Can you work these out from the model? Positions are in its coordinate system, mm. A direction names the side the tool comes from. Coordinates: 2 decimals unless noted, no trailing zeros. Loops run counter-clockwise (first coordinate to the right, second up) from the corner with the lowest first, then second, coordinate; pieces in that order, holes last. Notation, with made-up numbers: (34, -22.75) -> (60, -22.75) arc R17 cw to (60, -14.75) -> close; hole circle Ø11 at (74.5, 62). An arc over 180 degrees is marked (long way). Put each result on its own line as item: value. Start each with the question number.
Item 1: Will these pins go through, and if not, where does the flat tip stop? P1, Ø1.5, axis at y = 5, z = -3, coming from the +X side; P2, Ø2.5, axis at x = 3, y = 5, coming from the +Z side; P3, Ø1, axis at x = 3.5, y = 4, coming from the -Z side.
Item 2: If we section it at D-D on z = -3.25: Please give me the cut outline in (x, y).
Item 3: If we section it at C-C on x = 0: Please give me the cut outline in (y, z), plus the area to 3 significant figures.
Item 4: For faces 1 (the flat face through (-4.3, 5, -3)), 2 (the flat face through (0, 4, 5)), 3 (the flat face through (-3.5, 7, -3.5)), 4 (the flat face through (4.3, 5, -3)), 5 (the flat face through (0, 4, -5)), which set-ups out of +Z, -Z, +X, -X, +Y, -Y let a thin tool reach every point of the face, with its end or its side?
Item 5: We'd pull the mould along Z, two halves only. Please class faces 6 (the flat face through (-5, 4, 0)), 7 (the flat face through (3, 5, -4.3)), 8 (the cylindrical face through (5.723, 1.972, -1.802)), 9 (the cylindrical face through (5, 2, 1)): pulls with the +Z half, pulls with the -Z half, needs draft (parallel to the pull), parting line crosses it, or undercut.
Item 6: If we section it at A-A on z = 0: Please give me the cut outline in (x, y).
Item 7: Please list where these lines run through material, in increasing order: L1, parallel to Y at x = -5.7, z = 0; L2, parallel to Z at x = 0, y = 1.6; L3, parallel to Y at x = 0.75, z = -5.25. Write a range as from..to.
Item 8: If we section it at B-B on y = 5: Please give me the cut outline in (x, z).
```python
from build123d import *

# Parameters (mm, degrees)
SKETCH1_R               = 6
SKETCH1_R_2             = 4.5
BOSS_EXTRUDE5_DEPTH     = 4
BOSS_EXTRUDE6_DEPTH     = 3
SKETCH4_R               = 1
CUT_EXTRUDE1_DEPTH      = 7
CUT_EXTRUDE1_DEPTH_BACK = 7


with BuildPart() as part:
    # Sketch1 → Boss-Extrude5 (new body)
    with BuildSketch(Plane(origin=(0, 0, 0), x_dir=(1, 0, 0), z_dir=(0, 1, 0))):
        Circle(SKETCH1_R)
        Circle(SKETCH1_R_2, mode=Mode.SUBTRACT)
    extrude(amount=BOSS_EXTRUDE5_DEPTH)

    # Sketch3 → Boss-Extrude6 (add)
    with BuildSketch(Plane(origin=(0, 4, 0), x_dir=(1, 0, 0), z_dir=(0, 1, 0))):
        with BuildLine():
            Line((1.326649916, 4.3), (4.3, 4.3))
            Line((4.3, 4.3), (4.3, 1.326649916))
            ThreePointArc((4.3, 1.326649916), (3.181980515, 3.181980515), (1.326649916, 4.3))
        make_face()
        with BuildLine():
            Line((-4.3, -4.3), (-1.326649916, -4.3))
            ThreePointArc((-1.326649916, -4.3), (-3.181980515, -3.181980515), (-4.3, -1.326649916))
            Line((-4.3, -1.326649916), (-4.3, -4.3))
        make_face()
        with BuildLine():
            Line((-4.3, 4.3), (-1.326649916, 4.3))
            ThreePointArc((-1.326649916, 4.3), (-3.181980515, 3.181980515), (-4.3, 1.326649916))
            Line((-4.3, 1.326649916), (-4.3, 4.3))
        make_face()
        with BuildLine():
            Line((4.3, -4.3), (4.3, -1.326649916))
            ThreePointArc((4.3, -1.326649916), (3.181980515, -3.181980515), (1.326649916, -4.3))
            Line((1.326649916, -4.3), (4.3, -4.3))
        make_face()
    extrude(amount=BOSS_EXTRUDE6_DEPTH)

    # Sketch4 → Cut-Extrude1 (cut, two sides)
    with BuildSketch(Plane(origin=(0, 0, 0), x_dir=(0, 0, -1), z_dir=(1, 0, 0))) as cut_extrude1_sk:
        with Locations((0, 2)):
            Circle(SKETCH4_R)
    extrude(amount=CUT_EXTRUDE1_DEPTH, mode=Mode.SUBTRACT)
    extrude(cut_extrude1_sk.sketch, amount=-CUT_EXTRUDE1_DEPTH_BACK, mode=Mode.SUBTRACT)


solid = part.part
```
Solutions:
1. P1: x = 4.3
1. P2: z = 5.56
1. P3: z = -5.2
2. outline: (-5.04, 0) -> (-3.11, 0) -> (-3.11, 7) -> (-4.3, 7) -> (-4.3, 4) -> (-5.04, 4) -> close; (3.11, 0) -> (5.04, 0) -> (5.04, 4) -> (4.3, 4) -> (4.3, 7) -> (3.11, 7) -> close
3. outline: (0, -6) -> (4, -6) -> (4, -4.5) -> (0, -4.5) -> close; (0, 4.5) -> (4, 4.5) -> (4, 6) -> (0, 6) -> close
3. area: 12.0 mm^2
4. face 1: +Z, -Z, -X, +Y
4. face 2: +Z, +X, -X, +Y
4. face 3: +Z, -Z, +X, -X, +Y
4. face 4: +Z, -Z, +X, +Y
4. face 5: -Z, +X, -X, +Y
5. face 6: needs draft
5. face 7: pulls with the -Z half
5. face 8: parting line crosses it
5. face 9: undercut
6. outline: (-6, 0) -> (-4.5, 0) -> (-4.5, 1) -> (-6, 1) -> close; (-6, 3) -> (-4.5, 3) -> (-4.5, 4) -> (-6, 4) -> close; (4.5, 0) -> (6, 0) -> (6, 1) -> (4.5, 1) -> close; (4.5, 3) -> (6, 3) -> (6, 4) -> (4.5, 4) -> close
7. L1: 0..1, 3..4
7. L2: -6..-4.5, 4.5..6
7. L3: 0..4
8. outline: (-4.3, -4.3) -> (-1.33, -4.3) arc R4.5 cw to (-4.3, -1.33) -> close; (-4.3, 1.33) arc R4.5 cw to (-1.33, 4.3) -> (-4.3, 4.3) -> close; (1.33, -4.3) -> (4.3, -4.3) -> (4.3, -1.33) arc R4.5 cw to start; (1.33, 4.3) arc R4.5 cw to (4.3, 1.33) -> (4.3, 4.3) -> close
